CAD build for the part. Positions are in the model's coordinates, mm. Round coordinates to 2 decimals unless told otherwise and drop trailing zeros. Write each loop counter-clockwise with the first axis right and the second up, starting at its lowest first coordinate (ties: lowest second). Pieces come first, ordered by that corner, then holes. Notation, with made-up numbers: (80.5, 32) - (102.5, 32) arc R12 ccw to (102.5, 55) - close; hole circle Ø2 at (46, 72). An arc over 180 degrees is marked (long way). Use one line per item in the form item = value. Start each with the question number.
Item 1: Band-saw the part on C-C, the plane z = 4.25. List the corners of the cut face in (x, y) (3 decimals), and give its area (3 significant figures).
Item 2: Band-saw the part on B-B, the plane y = 28. List the corners of the cut face in (x, z).
Item 3: Pin check, flat tips, straight feed: pin 1 (6.5 mm diameter, centred on x = 9.271, y = -15.875, fed in from +Z); pin 2 (1.5 mm diameter, centred on x = -2, y = 27.5, fed in from +Z). Stop position of each tip, or through.
Item 4: Drill centre lines: L1, parallel to Y at x = -9, z = 0.5; L2, parallel to X at y = 10, z = 1; L3, parallel to Y at x = -2, z = 1.5. Where is each one in solid material? Low to high.
Item 5: Band-saw the part on A-A, the plane y = 10.5. List the corners of the cut face in (x, z).
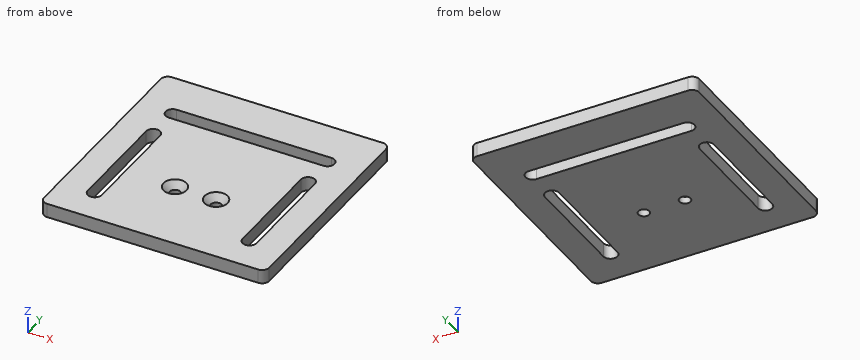
from build123d import *

# Parameters (mm, degrees)
F0_W           = 101.6
F0_H           = 101.6
F1_DEPTH       = 6.35
F3_D           = 4.9784
F3_CSINK_D     = 10.4394
F3_CSINK_ANGLE = 82
F4_R           = 3.175


with BuildPart() as f1:
    # F0 (on Top) → F1 (new body)
    with BuildSketch(Plane.XY):
        Rectangle(F0_W, F0_H)
        with BuildLine():
            Line((-38.1, -34.925), (-38.1, 12.7))
            ThreePointArc((-38.1, 12.7), (-34.925, 15.875), (-31.75, 12.7))
            Line((-31.75, 12.7), (-31.75, -34.925))
            ThreePointArc((-31.75, -34.925), (-34.925, -38.1), (-38.1, -34.925))
        make_face(mode=Mode.SUBTRACT)
        with BuildLine():
            Line((31.75, -34.925), (31.75, 12.7))
            ThreePointArc((31.75, 12.7), (34.925, 15.875), (38.1, 12.7))
            Line((38.1, 12.7), (38.1, -34.925))
            ThreePointArc((38.1, -34.925), (34.925, -38.1), (31.75, -34.925))
        make_face(mode=Mode.SUBTRACT)
        with BuildLine():
            Line((34.925, 25.4), (-34.925, 25.4))
            ThreePointArc((-34.925, 25.4), (-38.1, 28.575), (-34.925, 31.75))
            Line((-34.925, 31.75), (34.925, 31.75))
            ThreePointArc((34.925, 31.75), (38.1, 28.575), (34.925, 25.4))
        make_face(mode=Mode.SUBTRACT)
    extrude(amount=F1_DEPTH)

    # F3 (through all)
    with Locations(Plane.XY.offset(6.35)):
        with Locations((-9.271, -15.875), (9.271, -15.875)):
            CounterSinkHole(F3_D / 2, F3_CSINK_D / 2, counter_sink_angle=F3_CSINK_ANGLE)

    # F4
    f4_edges = [f1.edges().sort_by_distance(p)[0] for p in [
        (-50.8, -50.8, 3.175),
        (50.8, -50.8, 3.175),
        (-50.8, 50.8, 3.175),
        (50.8, 50.8, 3.175),
    ]]
    fillet(f4_edges, radius=F4_R)


solid = f1.part
Determined:
q1.outline = (-50.8, -47.625) arc R3.175 ccw to (-47.625, -50.8) - (47.625, -50.8) arc R3.175 ccw to (50.8, -47.625) - (50.8, 47.625) arc R3.175 ccw to (47.625, 50.8) - (-47.625, 50.8) arc R3.175 ccw to (-50.8, 47.625) - close; hole (-38.1, -34.925) arc R3.175 ccw to (-31.75, -34.925) - (-31.75, 12.7) arc R3.175 ccw to (-38.1, 12.7) - close; hole (-34.925, 25.4) - (34.925, 25.4) arc R3.175 ccw to (34.925, 31.75) - (-34.925, 31.75) arc R3.175 ccw to start; hole circle Ø6.788 at (-9.271, -15.875); hole circle Ø6.788 at (9.271, -15.875); hole (31.75, -34.925) arc R3.175 ccw to (38.1, -34.925) - (38.1, 12.7) arc R3.175 ccw to (31.75, 12.7) - close
q1.area = 9,100 mm²
q2.outline = (-50.8, 0) - (-38.05, 0) - (-38.05, 6.35) - (-50.8, 6.35) - close; (38.05, 0) - (50.8, 0) - (50.8, 6.35) - (38.05, 6.35) - close
q3.pin_1 = 4.08
q3.pin_2 = through
q4.L1 = -50.8 to -18.35, -13.4 to 25.4, 31.75 to 50.8
q4.L2 = -50.8 to -38.1, -31.75 to 31.75, 38.1 to 50.8
q4.L3 = -50.8 to 25.4, 31.75 to 50.8
q5.outline = (-50.8, 0) - (-38.1, 0) - (-38.1, 6.35) - (-50.8, 6.35) - close; (-31.75, 0) - (31.75, 0) - (31.75, 6.35) - (-31.75, 6.35) - close; (38.1, 0) - (50.8, 0) - (50.8, 6.35) - (38.1, 6.35) - close
